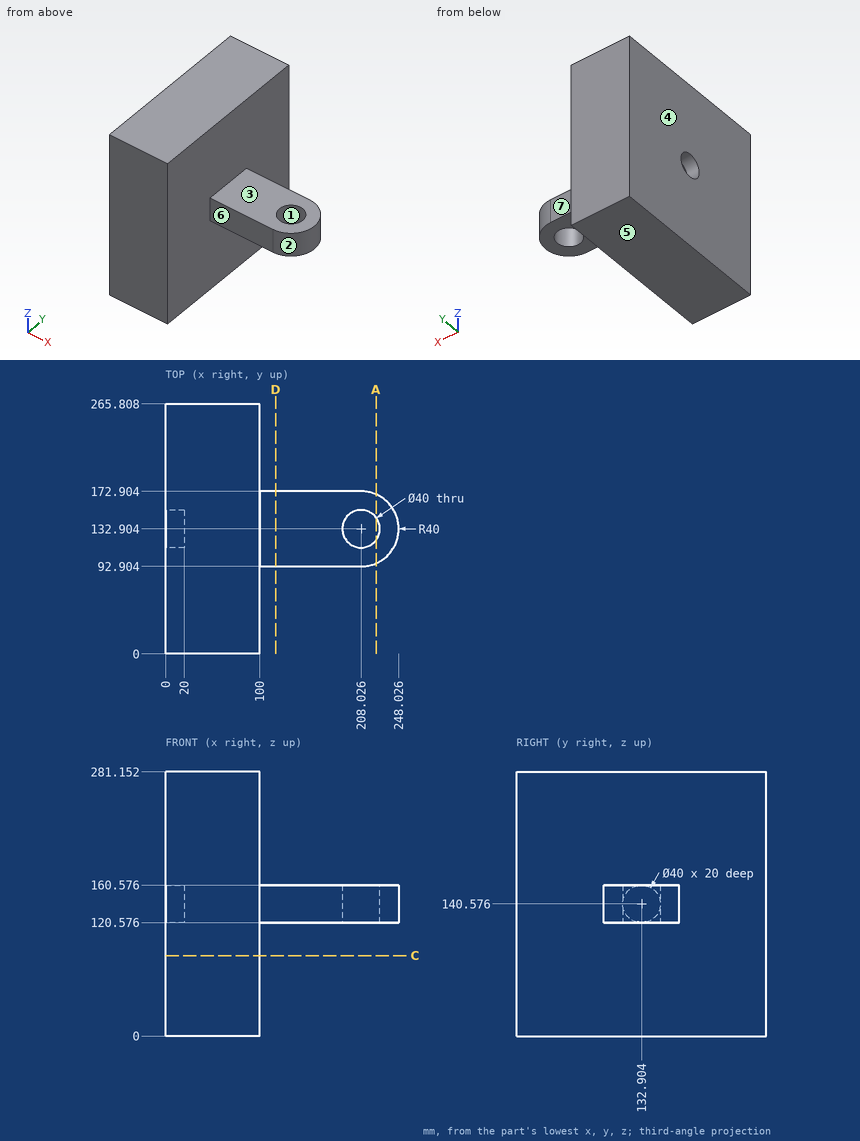
Study the drawing (mm; zero at the part's minimum x, y, z) and answer. A direction names the side the tool comes from. Give positions to 0.01 mm unless a question says otherwise; leave off trailing zeros. Write each loop counter-clockwise with the first axis right and the second up, starting at its lowest first coordinate (ties: lowest second). Pieces come first, ordered by that corner, then holes.
Item 1: Which of the six approach directions +Z, -Z, +X, -X, +Y, -Y give full straight-line access (tool end or side, diameter ignored) to the marked faces 5, 6 and 7?
Item 2: Determine the mould class of the marked faces 1, 2, 3 and 4 for opening direction X: released by +X, released by -X, zero draft, split by the parting line, or undercut.
Item 3: Section A-A, the plane x = 224 is taken. Write down the section's boundary in (y, z) (1 decimal), plus the area to 3 significant figures.
Item 4: Flat-ended cylindrical pins translate along their axes: P1, Ø2, axis at y = 75.5, z = 117, coming from the +X side; P2, Ø12, axis at y = 125, z = 141, coming from the -X side; P3, Ø20, axis at x = 159, z = 147.5, coming from the +Y side. Find the tip coordinate at first contact, or state that the pin passes through.
Item 5: Section D-D, the plane x = 117 is taken. Write down the section's boundary in (y, z) (1 decimal).
Item 6: Find the intervals of material crossed by line 1 along Z through (x, y) = (235, 108.5) (1 decimal); line 2 along X through (y, z) = (45.5, 258); line 3 along Y through (x, z) = (164.5, 122.5), in increasing order.
Item 7: Section C-C, the plane z = 85.5 is taken. Write down the section's boundary in (x, y).
Completed:
1. face 5: -Z, +X, -X, +Y, -Y
1. face 6: +Z, -Z, +X, -Y
1. face 7: +Z, -Z, +X, +Y
2. face 1: undercut
2. face 2: released by +X
2. face 3: zero draft
2. face 4: released by -X
3. outline: (96.2, 120.6) - (120.9, 120.6) - (120.9, 160.6) - (96.2, 160.6) - close; (144.9, 120.6) - (169.6, 120.6) - (169.6, 160.6) - (144.9, 160.6) - close
3. area: 1,970 mm2
4. P1: stops at x = 100
4. P2: stops at x = 20
4. P3: stops at y = 172.9
5. outline: (92.9, 120.6) - (172.9, 120.6) - (172.9, 160.6) - (92.9, 160.6) - close
6. line 1: z = 120.6 to 160.6
6. line 2: x = 0 to 100
6. line 3: y = 92.9 to 172.9
7. outline: (0, 0) - (100, 0) - (100, 265.81) - (0, 265.81) - close
